Read the model definition and answer for the solid it produces. Units are mm, in the model's axes. Coordinates: 2 decimals unless noted, no trailing zeros. Loops run counter-clockwise (first coordinate to the right, second up) from the corner with the lowest first, then second, coordinate; pieces in that order, holes last. Notation, with made-up numbers: (78.25, 21) -> (125.25, 21) arc R28 cw to (125.25, 55) -> close; hole circle Ø5 at (15, -29). An arc over 180 degrees is marked (long way). Answer in a Markdown table with one row per item.
Autodesk Inventor part; units mm, degrees
sketch "Эскиз1" plane through (0, 0, 0) normal (0, 1, 0) x (-1, 0, 0)
  line L0 (-2.8868, 0) -> (-1.4434, 2.5)
  line L1 (-1.4434, 2.5) -> (1.4434, 2.5)
  line L2 (1.4434, 2.5) -> (2.8868, 0)
  line L3 (2.8868, 0) -> (1.4434, -2.5)
  line L4 (1.4434, -2.5) -> (-1.4434, -2.5)
  line L5 (-1.4434, -2.5) -> (-2.8868, 0)
  circle A0 centre (0, 0) radius 1.5
  dimension "d0" = 5
  dimension "d2" = 3
extrude "Выдавливание1" add sketch "Эскиз1" along normal mid plane 8
properties part number "Стойка"
1. A cutting plane is placed at D-D on z = 2.05. Give the vertices of the cut face in (x, y), and give its area (3 significant figures).
A:
| item | result |
|---|---|
| outline | (-1.7, -4) -> (1.7, -4) -> (1.7, 4) -> (-1.7, 4) -> close |
| area | 27.3 mm2 |
2. A cutting plane is placed at A-A on x = 0. Give the vertices of the cut face in (y, z).
A:
| item | result |
|---|---|
| outline | (-4, -2.5) -> (4, -2.5) -> (4, -1.5) -> (-4, -1.5) -> close; (-4, 1.5) -> (4, 1.5) -> (4, 2.5) -> (-4, 2.5) -> close |
3. The mould has two halves that part along Z. Classify faces 1 (the flat face through (-2.175, -0.056, -1.233)), 2 (the flat face through (-1.24, 4, 1.15)), 3 (the flat face through (-2.155, -0.056, 1.267)), 4 (the cylindrical face through (1.5, -0.06, -0.07)): pulls with the +Z half, pulls with the -Z half, needs draft (parallel to the pull), parting line crosses it, or undercut.
A:
| item | result |
|---|---|
| face 1 | pulls with the -Z half |
| face 2 | needs draft |
| face 3 | pulls with the +Z half |
| face 4 | undercut |
4. A cutting plane is placed at B-B on y = 0.75. Give the vertices of the cut face in (x, z), and give its area (3 significant figures).
A:
| item | result |
|---|---|
| outline | (-2.89, 0) -> (-1.44, -2.5) -> (1.44, -2.5) -> (2.89, 0) -> (1.44, 2.5) -> (-1.44, 2.5) -> close; hole circle Ø3 at (0, 0) |
| area | 14.6 mm2 |
5. A cutting plane is placed at C-C on z = 1. Give the vertices of the cut face in (x, y), and give its area (3 significant figures).
A:
| item | result |
|---|---|
| outline | (-2.31, -4) -> (-1.12, -4) -> (-1.12, 4) -> (-2.31, 4) -> close; (1.12, -4) -> (2.31, -4) -> (2.31, 4) -> (1.12, 4) -> close |
| area | 19.1 mm2 |
6. Find the intervals of material crossed by probe 1 along Z at (x, y) = (0, -1.25); probe 2 along Z at (x, y) = (-0.65, -0.25); probe 3 along X at (y, z) = (-2.75, 1.1), in increasing order.
A:
| item | result |
|---|---|
| probe 1 | z = -2.5 to -1.5, 1.5 to 2.5 |
| probe 2 | z = -2.5 to -1.35, 1.35 to 2.5 |
| probe 3 | x = -2.25 to -1.02, 1.02 to 2.25 |
7. Given pin 1 Ø1 at (x, y) = (-2, 0) entering from -Z; pin 2 Ø3 at (x, z) = (-0.5, 0) entering from +Y; pin 3 Ø2.5 at (x, z) = (0, 0) entering from -Y; pin 4 Ø1.5 at (y, z) = (-1.5, 1.5) entering from +X, each flat-ended and moving along its own axis, determine where each tip first touches the part or whether it passes through.
A:
| item | result |
|---|---|
| pin 1 | stops at z = -2.4 |
| pin 2 | stops at y = 4 |
| pin 3 | passes through |
| pin 4 | stops at x = 2.45 |
